Build history of the part. All positions in model axes, mm. A direction names the side the tool comes from. Give positions to 0.01 mm unless a question says otherwise; leave off trailing zeros. Write each loop counter-clockwise with the first axis right and the second up, starting at its lowest first coordinate (ties: lowest second). Pieces come first, ordered by that corner, then holes. Notation, with made-up numbers: (-8, -19) -> (10, -19) arc R10 ccw to (10, -5) -> close; hole circle Ø9 at (80, 50). An arc over 180 degrees is marked (long way). Put each result on its own line as item: value. Start each with the question number.
Item 1: Drill centre lines: line 1 along X through (y, z) = (10.75, 0); line 2 along Y through (x, z) = (1, -3.5); line 3 along Y through (x, z) = (-5.5, -1.5). Where is each one in solid material? Low to high.
Item 2: Flat gauge pins, fed straight in: pin 1 Ø2 at (y, z) = (11, 4.5) entering from -X; pin 2 Ø2 at (x, y) = (7, 10.5) entering from +Z; pin 3 Ø1 at (x, y) = (-2, 17.5) entering from +Z; pin 4 Ø3 at (y, z) = (7.7, 7.04) entering from -X. Where does each tip first touch, or does it go through?
Item 3: Slice it at A-A, the plane z = -1. List the corners of the cut face in (x, y), plus the area to 3 significant figures.
Item 4: Slice it at B-B, the plane z = 0.65. List the corners of the cut face in (x, y), plus the area to 3 significant figures.
Item 5: Tool access for faces 4 (the cylindrical face through (8, 10, 0)), 5 (the cylindrical face through (-8, 10, 0)), 6 (the flat face through (0, 26, 0)), 7 (the cylindrical face through (0.1, 29.9, -3.9)): list every direction of +Z, -Z, +X, -X, +Y, -Y with a clear straight run to the whole face (end or side of a thin tool).
Item 6: Slice it at D-D, the plane z = 2.75. List the corners of the cut face in (x, y) (3 decimals).
Item 7: Two-plate mould, pull along Z, no slides. Class faces 1 (the cylindrical face through (3.18, 7.66, 5.49)), 2 (the flat face through (-5.79, 9.26, -5.97)), 3 (the flat face through (2, 13, 8)): pulls with the +Z half, pulls with the -Z half, needs draft (parallel to the pull), parting line crosses it, or undercut.
Item 8: Slice it at C-C, the plane y = 26. List the corners of the cut face in (x, z).
```python
from build123d import *

# Parameters (mm, degrees)
EXTRUDE_DEPTH                  = 20
EXTRUDE_ONTO_SKETCH_ROLL_ANGLE = 90
SKETCH001_R                    = 5
POCKET_DEPTH                   = 14
POCKET001_DEPTH                = 20.001
SKETCH003_R                    = 10
EXTRUDE001_DEPTH               = 8
SKETCH004_R                    = 10
POCKET002_DEPTH                = 8.001
POCKET003_DEPTH                = 8.001
SKETCH006_R                    = 1.55
POCKET004_DEPTH                = 9.676
POCKET004_DEPTH_BACK           = -10.326


with BuildPart() as pocket001:
    # Sketch as drawn → Extrude (new)
    with BuildSketch(Plane.XY):
        with BuildLine():
            Line((-4.618802, 8), (4.618805, 8))
            Line((4.618805, 8), (6.928207, 3.999994))
            ThreePointArc((6.928203, -4), (8, -3e-06), (6.928207, 3.999994))
            Line((4.618802, -8), (6.928203, -4))
            Line((-4.618805, -8), (4.618802, -8))
            Line((-6.928208, -3.999992), (-4.618805, -8))
            ThreePointArc((-6.928205, 3.999998), (-8, 3e-06), (-6.928208, -3.999992))
            Line((-4.618802, 8), (-6.928205, 3.999998))
        make_face()
    extrude(amount=-EXTRUDE_DEPTH)


with BuildPart() as pocket001_1:
    # Extrude onto Sketch roll: moved
    add(pocket001.part.rotate(Axis((0, 0, 0), (1, 0, 0)), EXTRUDE_ONTO_SKETCH_ROLL_ANGLE))


with BuildPart() as pocket001_2:
    # Extrude onto Sketch placement: moved
    add(pocket001_1.part)

    # Sketch001 → Pocket (cut)
    with BuildSketch(Plane.XZ):
        Circle(SKETCH001_R)
    extrude(amount=-POCKET_DEPTH, mode=Mode.SUBTRACT)

    # Sketch002 → Pocket001 (cut, through all)
    with BuildSketch(Plane(origin=(0, 20, 0), x_dir=(-1, 0, 0), z_dir=(0, 1, 0))):
        with BuildLine():
            ThreePointArc((-0.325, 1.212917), (0, 0), (0.325, 1.212917))
            Line((0.325, 8), (0.325, 1.212917))
            Line((-0.325, 8), (0.325, 8))
            Line((-0.325, 8), (-0.325, 1.212917))
        make_face()
    extrude(amount=-POCKET001_DEPTH, mode=Mode.SUBTRACT)


with BuildPart() as pocket004:
    # Sketch003 → Extrude001 (new body)
    with BuildSketch(Plane(origin=(0, 0, -8), x_dir=(1, 0, 0), z_dir=(0, 0, -1))):
        with Locations((0, -26)):
            Circle(SKETCH003_R)
    extrude(amount=-EXTRUDE001_DEPTH)

    # Fusion: union Pocket001
    add(pocket001_2.part)

    # Sketch004 → Pocket002 (cut, through all)
    with BuildSketch(Plane.XY):
        with Locations((0, 26)):
            Circle(SKETCH004_R)
    extrude(amount=POCKET002_DEPTH, mode=Mode.SUBTRACT)

    # Sketch005 → Pocket003 (cut, through all)
    with BuildSketch(Plane.XY):
        with BuildLine():
            ThreePointArc((3.194693, 28.236948), (0, 29.9), (-3.194693, 28.236948))
            ThreePointArc((-5.734064, 30.015035), (-5.353422, 27.856306), (-3.194693, 28.236948))
            ThreePointArc((5.734064, 30.015035), (0, 33), (-5.734064, 30.015035))
            ThreePointArc((3.194693, 28.236948), (5.353422, 27.856306), (5.734064, 30.015035))
        make_face()
        with BuildLine():
            ThreePointArc((-3.194693, 23.763052), (0, 22.1), (3.194693, 23.763052))
            ThreePointArc((5.734064, 21.984965), (5.353422, 24.143694), (3.194693, 23.763052))
            ThreePointArc((-5.734064, 21.984965), (0, 19), (5.734064, 21.984965))
            ThreePointArc((-3.194693, 23.763052), (-5.353422, 24.143694), (-5.734064, 21.984965))
        make_face()
    extrude(amount=-POCKET003_DEPTH, mode=Mode.SUBTRACT)

    # Sketch006 → Pocket004 (cut, two sides)
    with BuildSketch(Plane.YZ.offset(-0.325)) as pocket004_sk:
        with Locations((7.70394, 7.039426)):
            Circle(SKETCH006_R)
    extrude(amount=-POCKET004_DEPTH, mode=Mode.SUBTRACT)
    extrude(pocket004_sk.sketch, amount=-POCKET004_DEPTH_BACK, mode=Mode.SUBTRACT)


solid = pocket004.part
```
Values follow:
1. line 1: -8 to -5, 5 to 8
1. line 2: 14 to 19.07, 22.23 to 29.77, 32.93 to 35.95
1. line 3: 0 to 21.67, 24.03 to 27.97, 30.33 to 34.35
2. pin 1: x = -7.19
2. pin 2: z = 5.61
2. pin 3: z = 0
2. pin 4: through
3. outline: (-7.94, 0) -> (-4.9, 0) -> (-4.9, 14) -> (4.9, 14) -> (4.9, 0) -> (7.94, 0) -> (7.94, 19.92) arc R10 ccw (long way) to (-7.94, 19.92) -> close; hole (-5.73, 21.98) arc R7 ccw to (5.73, 21.98) arc R1.55 ccw to (3.19, 23.76) arc R3.9 cw to (-3.19, 23.76) arc R1.55 ccw to start; hole (-5.73, 30.02) arc R1.55 ccw to (-3.19, 28.24) arc R3.9 cw to (3.19, 28.24) arc R1.55 ccw to (5.73, 30.02) arc R7 ccw to start
3. area: 370 mm2
4. outline: (-7.97, 0) -> (-4.96, 0) -> (-4.96, 14) -> (-0.65, 14) -> (-0.65, 16.02) arc R10 cw to (-7.97, 19.96) -> close; (0.65, 14) -> (4.96, 14) -> (4.96, 0) -> (7.97, 0) -> (7.97, 19.96) arc R10 cw to (0.65, 16.02) -> close
4. area: 133 mm2
5. face 4: +X, -Y
5. face 5: -X, -Y
5. face 6: +Z, +Y
5. face 7: +Z, -Z
6. outline: (-7.512, 0) -> (-4.176, 0) -> (-4.176, 14) -> (-0.325, 14) -> (-0.325, 16.005) arc R10 cw to (-7.512, 19.4) -> close; (0.325, 14) -> (4.176, 14) -> (4.176, 0) -> (7.512, 0) -> (7.512, 19.4) arc R10 cw to (0.325, 16.005) -> close
7. face 1: undercut
7. face 2: pulls with the -Z half
7. face 3: pulls with the +Z half
8. outline: (-10, -8) -> (10, -8) -> (10, 0) -> (-10, 0) -> close
